```python
from build123d import *

# Parameters (mm, degrees)
BOSS_EXTRUDE1_DEPTH = 25
CUT_EXTRUDE2_DEPTH  = 26
BOSS_EXTRUDE2_DEPTH = 0.4


with BuildPart() as part:
    # Sketch1 → Boss-Extrude1 (new body)
    with BuildSketch(Plane(origin=(0, 0, 0), x_dir=(1, 0, 0), z_dir=(0, 1, 0))):
        with BuildLine():
            ThreePointArc((1.451818925, -34.068556857), (1.641248992, -34.346908706), (1.964225605, -34.442038138))
            ThreePointArc((1.964225605, -34.442038138), (26.591847487, -21.978073076), (34.198225299, 4.555174015))
            ThreePointArc((34.198225299, 4.555174015), (23.590291339, 25.176355888), (2.324135821, 34.423627607))
            ThreePointArc((2.324135821, 34.423627607), (1.751838249, 34.289058819), (1.354061739, 33.856153382))
            ThreePointArc((1.354061739, 33.856153382), (0, 33.001534515), (-1.354061739, 33.856153382))
            ThreePointArc((-1.354061739, 33.856153382), (-1.751838249, 34.289058819), (-2.324135821, 34.423627607))
            ThreePointArc((-2.324135821, 34.423627607), (-23.590291339, 25.176355888), (-34.198225299, 4.555174015))
            ThreePointArc((-34.198225299, 4.555174015), (-26.591847487, -21.978073076), (-1.964225605, -34.442038138))
            ThreePointArc((-1.964225605, -34.442038138), (-1.641248992, -34.346908706), (-1.451818925, -34.068556857))
            ThreePointArc((-1.451818925, -34.068556857), (0, -32.945679925), (1.451818925, -34.068556857))
        make_face()
        with BuildLine():
            Line((-2.417, 3.787737139), (0, 3.787737139))
            Line((0, 3.787737139), (2.417, 3.787737139))
            ThreePointArc((2.417, 3.787737139), (0, -4.489512172), (-2.417, 3.787737139))
        make_face(mode=Mode.SUBTRACT)
    extrude(amount=BOSS_EXTRUDE1_DEPTH)

    # Sketch2 → Cut-Extrude2 (cut, through all)
    with BuildSketch(Plane(origin=(0, 0, 0), x_dir=(1, 0, 0), z_dir=(0, 1, 0))):
        with BuildLine():
            ThreePointArc((-29.910714286, -2.312827473), (-21.213203436, -21.213203436), (-2.312827473, -29.910714286))
            ThreePointArc((-2.312827473, -29.910714286), (-1.448498888, -29.786346067), (-0.719546325, -29.305555556))
            ThreePointArc((-0.719546325, -29.305555556), (0, -29), (0.719546325, -29.305555556))
            ThreePointArc((0.719546325, -29.305555556), (1.448498888, -29.786346067), (2.312827473, -29.910714286))
            ThreePointArc((2.312827473, -29.910714286), (21.213203436, -21.213203436), (29.910714286, -2.312827473))
            ThreePointArc((29.910714286, -2.312827473), (29.786346067, -1.448498888), (29.305555556, -0.719546325))
            ThreePointArc((29.305555556, -0.719546325), (29, 0), (29.305555556, 0.719546325))
            ThreePointArc((29.305555556, 0.719546325), (29.786346067, 1.448498888), (29.910714286, 2.312827473))
            ThreePointArc((29.910714286, 2.312827473), (21.213203436, 21.213203436), (2.312827473, 29.910714286))
            ThreePointArc((2.312827473, 29.910714286), (1.448498888, 29.786346067), (0.719546325, 29.305555556))
            ThreePointArc((0.719546325, 29.305555556), (0, 29), (-0.719546325, 29.305555556))
            ThreePointArc((-0.719546325, 29.305555556), (-1.448498888, 29.786346067), (-2.312827473, 29.910714286))
            ThreePointArc((-2.312827473, 29.910714286), (-21.213203436, 21.213203436), (-29.910714286, 2.312827473))
            ThreePointArc((-29.910714286, 2.312827473), (-29.786346067, 1.448498888), (-29.305555556, 0.719546325))
            ThreePointArc((-29.305555556, 0.719546325), (-29, 0), (-29.305555556, -0.719546325))
            ThreePointArc((-29.305555556, -0.719546325), (-29.786346067, -1.448498888), (-29.910714286, -2.312827473))
        make_face()
    extrude(amount=CUT_EXTRUDE2_DEPTH, mode=Mode.SUBTRACT)

    # Sketch2<2> → Boss-Extrude2 (add)
    with BuildSketch(Plane(origin=(0, 0, 0), x_dir=(1, 0, 0), z_dir=(0, 1, 0))):
        with BuildLine():
            ThreePointArc((-29.910714286, -2.312827473), (-21.213203436, -21.213203436), (-2.312827473, -29.910714286))
            ThreePointArc((-2.312827473, -29.910714286), (-1.448498888, -29.786346067), (-0.719546325, -29.305555556))
            ThreePointArc((-0.719546325, -29.305555556), (0, -29), (0.719546325, -29.305555556))
            ThreePointArc((0.719546325, -29.305555556), (1.448498888, -29.786346067), (2.312827473, -29.910714286))
            ThreePointArc((2.312827473, -29.910714286), (21.213203436, -21.213203436), (29.910714286, -2.312827473))
            ThreePointArc((29.910714286, -2.312827473), (29.786346067, -1.448498888), (29.305555556, -0.719546325))
            ThreePointArc((29.305555556, -0.719546325), (29, 0), (29.305555556, 0.719546325))
            ThreePointArc((29.305555556, 0.719546325), (29.786346067, 1.448498888), (29.910714286, 2.312827473))
            ThreePointArc((29.910714286, 2.312827473), (21.213203436, 21.213203436), (2.312827473, 29.910714286))
            ThreePointArc((2.312827473, 29.910714286), (1.448498888, 29.786346067), (0.719546325, 29.305555556))
            ThreePointArc((0.719546325, 29.305555556), (0, 29), (-0.719546325, 29.305555556))
            ThreePointArc((-0.719546325, 29.305555556), (-1.448498888, 29.786346067), (-2.312827473, 29.910714286))
            ThreePointArc((-2.312827473, 29.910714286), (-21.213203436, 21.213203436), (-29.910714286, 2.312827473))
            ThreePointArc((-29.910714286, 2.312827473), (-29.786346067, 1.448498888), (-29.305555556, 0.719546325))
            ThreePointArc((-29.305555556, 0.719546325), (-29, 0), (-29.305555556, -0.719546325))
            ThreePointArc((-29.305555556, -0.719546325), (-29.786346067, -1.448498888), (-29.910714286, -2.312827473))
        make_face()
    extrude(amount=BOSS_EXTRUDE2_DEPTH)


solid = part.part
```
Verification items for the finished model (mm, model axes). A direction names the side the tool comes from. Coordinates: 2 decimals unless noted, no trailing zeros. Write each loop counter-clockwise with the first axis right and the second up, starting at its lowest first coordinate (ties: lowest second). Pieces come first, ordered by that corner, then holes. Notation, with made-up numbers: M -16.75,54.25 L 23.25,54.25 A24 cw 23.25,73.25 Z; hole C 13,32 d11. An arc over 180 degrees is marked long. One line per item, written item: value.
Item 1: Section check C-C, the plane z = -7. Record the boundary of the cut face in (x, y).
Check sheet entries:
outline: M -33.78,0 L 33.78,0 L 33.78,25 L 29.17,25 L 29.17,0.4 L -29.17,0.4 L -29.17,25 L -33.78,25 Z
Item 2: Section check A-A, the plane y = 21.5. Record the boundary of the cut face in (x, z), plus the area to 3 significant figures.
Check sheet entries:
outline: M -2.32,-34.42 A1 ccw -1.35,-33.86 A1.5 cw 1.35,-33.86 A1 ccw 2.32,-34.42 A34.5 ccw 1.96,34.44 A0.5 ccw 1.45,34.07 A1.5 cw -1.45,34.07 A0.5 ccw -1.96,34.44 A34.5 ccw Z; hole M -29.91,-2.31 A30 ccw -2.31,-29.91 A2 ccw -0.72,-29.31 A1 cw 0.72,-29.31 A2 ccw 2.31,-29.91 A30 ccw 29.91,-2.31 A2 ccw 29.31,-0.72 A1 cw 29.31,0.72 A2 ccw 29.91,2.31 A30 ccw 2.31,29.91 A2 ccw 0.72,29.31 A1 cw -0.72,29.31 A2 ccw -2.31,29.91 A30 ccw -29.91,2.31 A2 ccw -29.31,0.72 A1 cw -29.31,-0.72 A2 ccw Z
area: 912 mm^2
Item 3: Scan lines: line 1 along Y through (x, z) = (26.5, -9); line 2 along X through (y, z) = (12, -6.5); line 3 along X through (y, z) = (5, 26.5). Record each from-to range of solid material in increasing order.
Check sheet entries:
line 1: y = 0 to 0.4
line 2: x = -33.88 to -29.29, 29.29 to 33.88
line 3: x = -22.09 to -14.06, 14.06 to 22.09
Item 4: Gauge pin test, flat ends, axial feed: pin 1 Ø6 at (x, y) = (7, 8) entering from -Z; pin 2 Ø10 at (x, y) = (-12.5, 4) entering from +Z; pin 3 Ø4 at (x, z) = (23.5, 9) entering from +Y. Record the tip position at first contact, or that the pin passes through.
Check sheet entries:
pin 1: stops at z = -34.27
pin 2: stops at z = 33.67
pin 3: stops at y = 0.4
Item 5: Access from +Z, -Z, +X, -X, +Y, -Y to the whole of each face (thin tool, end or side, straight path). Record for faces 1 (the flat face through (0, 0.4, 0)), 2 (the cylindrical face through (-0.028, 12.325, 32.946)).
Check sheet entries:
face 1: +Y
face 2: +Z, +Y, -Y
Item 6: Section check B-B, the plane x = 14. Record the boundary of the cut face in (y, z), plus the area to 3 significant figures.
Check sheet entries:
outline: M 0,-31.53 L 25,-31.53 L 25,-26.53 L 0.4,-26.53 L 0.4,26.53 L 25,26.53 L 25,31.53 L 0,31.53 Z
area: 271 mm^2
